Solid Edge part; units mm, degrees
sketch "Sketch1" plane through (0, 0, 0) normal (0, 0, 1) x (1, 0, 0)
  line L0 (-84.5, -50) -> (84.5, -50)
  line L1 (84.5, -50) -> (84.5, 50)
  line L2 (84.5, 50) -> (-84.5, 50)
  line L3 (-84.5, 50) -> (-84.5, -50)
  dimension "D1" = 84.5
  dimension "D2" = 84.5
extrude "Protrusion1" add sketch "Sketch1" along normal blind 3
sketch "Sketch2" plane through (0, -50, 1.5) normal (0, -1, 0) x (1, 0, 0)
  line L0 (-84.5, 1.5) -> (-84.5, 7.5)
  line L1 (-84.5, 7.5) -> (-78.5, 7.5)
  line L2 (-78.5, 7.5) -> (-78.5, 4.75)
  line L3 (-78.5, 4.75) -> (-81.75, 4.75)
  line L4 (-81.75, 4.75) -> (-81.75, 1.5)
  line L5 (-81.75, 1.5) -> (-84.5, 1.5)
  line L6 (84.5, 1.5) -> (84.5, 7.5)
  line L7 (84.5, 7.5) -> (78.5, 7.5)
  line L8 (78.5, 7.5) -> (78.5, 4.75)
  line L9 (78.5, 4.75) -> (81.75, 4.75)
  line L10 (81.75, 4.75) -> (81.75, 1.5)
  line L11 (81.75, 1.5) -> (84.5, 1.5)
extrude "Extrusionsausschnitt_1" add sketch "Sketch2" against normal blind 100
sketch "Sketch3" plane through (0, 50, 4.5) normal (0, 1, 0) x (-1, 0, 0)
  line L0 (84.5, -4.5) -> (-84.5, -4.5)
  line L1 (-84.5, -4.5) -> (-84.5, 4.5)
  line L2 (-84.5, 4.5) -> (84.5, 4.5)
  line L3 (84.5, 4.5) -> (84.5, -4.5)
extrude "Extrusionsausprägung_3" add sketch "Sketch3" against normal blind 3
sketch "Sketch4" plane through (84.5, 0, 4.5) normal (1, 0, 0) x (0, 1, 0)
  line L0 (-30, 4.5) -> (-16.4953, 38.1099)
  line L1 (10, 4.5) -> (-3.5047, 38.1099)
  line L2 (-30, 4.5) -> (10, 4.5)
  arc A0 (-16.4953, 38.1099) -> (-3.5047, 38.1099) centre (-10, 35.5) cw
  dimension "D1" = 30
extrude "Extrusionsausprägung_4" add sketch "Sketch4" against normal blind 6
hole "Bohrung_2" at (78.5, -10, 40) direction (1, 0, 0) diameter 5.8 end up to next countersink diameter 10.4 countersink angle 90
sketch "Sketch5" plane through (84.5, 0, 23.5) normal (1, 0, 0) x (0, 1, 0)
  line L0 (13.7478, -14.5) -> (20, -14.5)
  line L1 (20, -14.5) -> (20, 0.5)
  line L2 (20, 0.5) -> (13.7478, 0.5)
  line L3 (13.7478, 0.5) -> (13.7478, -14.5)
  dimension "D1" = 20
extrude "Extrusionsausprägung_5" add sketch "Sketch5" against normal blind 6 and the other way blind 10
Can you work these out from the model? Positions are in its coordinate system, mm. A direction names the side the tool comes from. Give positions to 0.01 mm unless a question says otherwise; leave off trailing zeros. Loops run counter-clockwise (first coordinate to the right, second up) from the corner with the lowest first, then second, coordinate; pieces in that order, holes last. Notation, with made-up numbers: M 69,30 L 108,30 A33 cw 108,58 Z; hole C 20,-3 d2. An arc over 180 degrees is marked long. One line per item, written item: value. Start each with the question number.
1) If I drill on line 1 (Z direction, x = 83, y = -10); line 2 (Y direction, x = 83.55, z = 40); line 3 (Z direction, x = -42, y = -8.5), over which ranges is the centre line in solid material (lowest first)? Write a range as [from, to].
2) On a 3-axis mill with a long thin cutter (end or side, diameter ignored), from which of +Z, -Z, +X, -X, +Y, -Y can I reach the whole of each face in a straight line? I mean faces 5 (the face through (90, 17, 9)), 6 (the face through (-81.75, -2, 5)), 7 (the face through (87, 13.748, 17)), 8 (the face through (81, -40, 9)). Say none if no direction works.
3) I'm going to push flat-ended pins straight in: pin 1 (12 mm diameter, centred on x = 70, y = 38.5, fed in from +Z); pin 2 (7.5 mm diameter, centred on x = 87.5, z = 15, fed in from +Y); pin 3 (1.4 mm diameter, centred on y = -13.5, z = 8, fed in from +X); pin 4 (3.5 mm diameter, centred on y = -10, z = 40, fed in from -X). Where does each tip first touch, or does it pass through?
4) Thinking about a two-plate mould opening in Z: for faces 1 (the face through (82, -10, 47)), 2 (the face through (82.624, -9.129, 42.766)), 3 (the face through (80.656, -11.166, 42.812)), 4 (the face through (-84.5, 1, 4)), which applies, +Z half, -Z half, draft (parallel to the pull), parting line (faces both ways), or undercut?
5) If we section it at D-D, the plane y = 39: Write out the boundary of the cut face in (x, z), and give its area (3 significant figures).
6) If we section it at A-A, the plane y = -10: Write out the boundary of the cut face in (x, z).
7) If we section it at B-B, the plane z = 20.5: Write out the boundary of the cut face in (x, y), and give its area (3 significant figures).
8) If we section it at C-C, the plane x = 47.5: Write out the boundary of the cut face in (y, z).
Completed:
1. line 1: z = [0, 37.1], [42.9, 47]
1. line 2: y = [-17.54, -12.9], [-7.1, -2.46]
1. line 3: z = [0, 3]
2. face 5: -Z, +X, +Y, -Y
2. face 6: -Y
2. face 7: +Z, +X, -X
2. face 8: +Z, +X, -X, -Y
3. pin 1: stops at z = 3
3. pin 2: stops at y = 20
3. pin 3: stops at x = 84.5
3. pin 4: passes through
4. face 1: +Z half
4. face 2: undercut
4. face 3: undercut
4. face 4: draft
5. outline: M -84.5,0 L 84.5,0 L 84.5,9 L 78.5,9 L 78.5,6.25 L 81.75,6.25 L 81.75,3 L -81.75,3 L -81.75,6.25 L -78.5,6.25 L -78.5,9 L -84.5,9 Z
5. area: 558 mm^2
6. outline: M -84.5,0 L 84.5,0 L 84.5,37.1 L 80.8,37.1 L 78.5,34.8 L 78.5,6.25 L 81.75,6.25 L 81.75,3 L -81.75,3 L -81.75,6.25 L -78.5,6.25 L -78.5,9 L -84.5,9 Z; M 78.5,45.2 L 80.8,42.9 L 84.5,42.9 L 84.5,47 L 78.5,47 Z
7. outline: M 78.5,-25.38 L 84.5,-25.38 L 84.5,5.38 L 78.5,5.38 Z; M 78.5,13.75 L 94.5,13.75 L 94.5,20 L 78.5,20 Z
7. area: 285 mm^2
8. outline: M -50,0 L 50,0 L 50,9 L 47,9 L 47,3 L -50,3 Z
